Design review of the part built by this model. Coordinates are the model's own, in mm. Coordinates: 2 decimals unless noted, no trailing zeros. Order: outer loops, then holes, each group sorted by start corner. A loop starts at its lowest first (then second) coordinate and runs counter-clockwise, first axis right, second up. Notation, with made-up numbers: (-17, 45) -> (-13, 45) arc R17 cw to (-13, 60) -> close; hole circle Ø4 at (-24, 39.5). An arc over 180 degrees is marked (long way). Write item = value, one per line.
```python
from build123d import *

# Parameters (mm, degrees)
SKETCH1_W               = 10
SKETCH1_H               = 40
BOSS_EXTRUDE1_DEPTH     = 700
CUT_EXTRUDE1_DEPTH      = 702.21323433
CUT_EXTRUDE1_DEPTH_BACK = 702.21323433
SKETCH2_W               = 5
SKETCH2_H               = 30
SKETCH3_R               = 2.5
CUT_EXTRUDE2_DEPTH      = 702.21323433


with BuildPart() as part:
    # Sketch1 → Boss-Extrude1 (new body)
    with BuildSketch(Plane.XY):
        with Locations((5, 20)):
            Rectangle(SKETCH1_W, SKETCH1_H)
    extrude(amount=BOSS_EXTRUDE1_DEPTH)

    # Sketch2 → Cut-Extrude1 (cut, two sides: drawn at the far end of the back side and taken through both)
    with BuildSketch(Plane.XY.offset(700).offset(-CUT_EXTRUDE1_DEPTH_BACK)):
        with Locations((2.5, 20)):
            Rectangle(SKETCH2_W, SKETCH2_H)
    extrude(amount=CUT_EXTRUDE1_DEPTH + CUT_EXTRUDE1_DEPTH_BACK, mode=Mode.SUBTRACT)

    # Sketch3 → Cut-Extrude2 (cut, through all)
    with BuildSketch(Plane(origin=(10, 0, 0), x_dir=(0, 0, -1), z_dir=(1, 0, 0))):
        with Locations((-693, 20)):
            Circle(SKETCH3_R)
        with Locations((-665, 20)):
            Circle(SKETCH3_R)
        with Locations((-633, 20)):
            Circle(SKETCH3_R)
        with Locations((-602, 20)):
            Circle(SKETCH3_R)
        with Locations((-570, 20)):
            Circle(SKETCH3_R)
        with Locations((-442, 20)):
            Circle(SKETCH3_R)
        with Locations((-283, 20)):
            Circle(SKETCH3_R)
        with Locations((-252, 20)):
            Circle(SKETCH3_R)
        with Locations((-123, 20)):
            Circle(SKETCH3_R)
        with Locations((-92, 20)):
            Circle(SKETCH3_R)
        with Locations((-59, 20)):
            Circle(SKETCH3_R)
        with Locations((-28, 20)):
            Circle(SKETCH3_R)
    extrude(amount=-CUT_EXTRUDE2_DEPTH, mode=Mode.SUBTRACT)


solid = part.part
```
(1) Insertion check: pin 1 (8 mm diameter, centred on y = 20, z = 633, fed in from +X); pin 2 (6 mm diameter, centred on y = 20, z = 59, fed in from -X). Each pin has a flat end and moves straight along its axis. Give the tip position at first contact, or say it passes through.
Report:
pin_1 = 10
pin_2 = 5
(2) We need section A-A (x = 2.25). Write out the cut boundary in (y, z).
Report:
outline = (0, 0) -> (5, 0) -> (5, 700) -> (0, 700) -> close; (35, 0) -> (40, 0) -> (40, 700) -> (35, 700) -> close
(3) We need section B-B (z = 193). Write out the cut boundary in (x, y).
Report:
outline = (0, 0) -> (10, 0) -> (10, 40) -> (0, 40) -> (0, 35) -> (5, 35) -> (5, 5) -> (0, 5) -> close
(4) The part is to be moulded in two halves that separate along Y. For faces 1 (the flat face through (10, 20, 345)), 2 (the flat face through (5, 20, 345)), say which applies: released by +Y, released by -Y, zero draft, split by the parting line, or undercut.
Report:
face_1 = zero draft
face_2 = undercut
(5) For L1, parallel to Y at x = 9.75, z = 602; L2, parallel to X at y = 27, z = 118.5; L3, parallel to Y at x = 2.75, z = 490, list the stretches that pass through material, from the lowest coordinate up.
Report:
L1 = 0 to 17.5, 22.5 to 40
L2 = 5 to 10
L3 = 0 to 5, 35 to 40
